Verification items for the finished model (mm, model axes). A direction names the side the tool comes from. Give positions to 0.01 mm unless a question says otherwise; leave off trailing zeros. Loops run counter-clockwise (first coordinate to the right, second up) from the corner with the lowest first, then second, coordinate; pieces in that order, holes last. Notation, with made-up numbers: (34.25, -9) - (87.25, -9) arc R21 cw to (87.25, 7) - close; hole circle Ø4 at (7, 86). An arc over 180 degrees is marked (long way). Use one line per item in the form item = value.
```python
from build123d import *

# Parameters (mm, degrees)
SKETCH068_R  = 1.7
PAD050_DEPTH = 100
SKETCH067_R  = 1.5
PAD049_DEPTH = 3
PAD048_DEPTH = 3


with BuildPart() as mountscrewcutouts:
    # Sketch068 → Pad050 (new body)
    with BuildSketch(Plane.XY):
        with Locations((28.75, 0)):
            Circle(SKETCH068_R)
        with Locations((18.75, 0)):
            Circle(SKETCH068_R)
    extrude(amount=-PAD050_DEPTH)


with BuildPart() as baseplate:
    # Sketch067 → Pad049 (new body)
    with BuildSketch(Plane(origin=(0, 0, -23), x_dir=(-1, 0, 0), z_dir=(0, 0, 1))):
        Polygon((-31.5, -4), (-31.5, 4), (-16.5, 7.5), (0, 7.5), (0, -7.5), (-16.5, -7.5), align=None)
        with Locations((-5, 3)):
            Circle(SKETCH067_R, mode=Mode.SUBTRACT)
        with Locations((-5, -3)):
            Circle(SKETCH067_R, mode=Mode.SUBTRACT)
    extrude(amount=-PAD049_DEPTH)


with BuildPart() as supportplate:
    # Sketch066 → Pad048 (new body)
    with BuildSketch(Plane(origin=(0, 0, -20), x_dir=(-1, 0, 0), z_dir=(0, 0, 1))):
        Polygon((-31.5, -4), (-31.5, 4), (-16.5, 7.5), (-16.5, -7.5), align=None)
    extrude(amount=-PAD048_DEPTH)

    # Fusion004017: union BasePlate
    add(baseplate.part)

    # Cut007017: cut MountScrewCutouts
    add(mountscrewcutouts.part, mode=Mode.SUBTRACT)


with BuildPart() as fusion004018:
    # Part__Mirroring001: instance of SupportPlate
    add(supportplate.part.mirror(Plane(origin=(0, 0, 0), x_dir=(0, -1, 0), z_dir=(1, 0, 0))))

    # Fusion004018: union SupportPlate
    add(supportplate.part)


solid = fusion004018.part
```
1. Tool access check on faces 5 (the flat face through (0, 0, -23)), 6 (the flat face through (-24, 0, -20)). Record the directions out of +Z, -Z, +X, -X, +Y, -Y that give a thin tool (end or side, any length) a straight path to the whole face; none if there is none.
Result set:
face_5 = +Z, +Y, -Y
face_6 = +Z, +X, -X, +Y, -Y
2. Section check B-B, the plane y = 3. Record the cut outline in (x, z).
Result set:
outline = (-31.5, -26) - (-6.5, -26) - (-6.5, -23) - (-16.5, -23) - (-16.5, -20) - (-31.5, -20) - close; (-3.5, -26) - (3.5, -26) - (3.5, -23) - (-3.5, -23) - close; (6.5, -26) - (31.5, -26) - (31.5, -20) - (16.5, -20) - (16.5, -23) - (6.5, -23) - close
3. Scan lines: probe 1 along X at (y, z) = (3, -24.15); probe 2 along X at (y, z) = (3, -20.7); probe 3 along Y at (x, z) = (4, -23.55). Record each from-to range of solid material in increasing order.
Result set:
probe_1 = -31.5 to -6.5, -3.5 to 3.5, 6.5 to 31.5
probe_2 = -31.5 to -16.5, 16.5 to 31.5
probe_3 = -7.5 to -4.12, -1.88 to 1.88, 4.12 to 7.5
4. Draft check along Y on faces 1 (the cylindrical face through (-20.3, -0.7, -23)), 2 (the flat face through (-16.5, 0, -21)), 3 (the flat face through (23.895, 5.774, -22.958)), 4 (the cylindrical face through (30.3, -0.7, -23)). Enter one of: released by +Y, released by -Y, zero draft, split by the parting line, or undercut.
Result set:
face_1 = undercut
face_2 = zero draft
face_3 = released by +Y
face_4 = undercut
5. Depth check by flat-ended pin: pin 1 Ø7.5 at (x, y) = (1.5, 1.5) entering from +Z. Enter the tip coordinate at first touch or a pass-through.
Result set:
pin_1 = -23
6. Section check C-C, the plane x = 5. Record the cut outline in (y, z), then the cut area to 3 significant figures.
Result set:
outline = (-7.5, -26) - (-4.5, -26) - (-4.5, -23) - (-7.5, -23) - close; (-1.5, -26) - (1.5, -26) - (1.5, -23) - (-1.5, -23) - close; (4.5, -26) - (7.5, -26) - (7.5, -23) - (4.5, -23) - close
area = 27.0 mm²
7. Section check D-D, the plane y = 0. Record the cut outline in (x, z), then the cut area to 3 significant figures.
Result set:
outline = (-31.5, -26) - (-30.45, -26) - (-30.45, -20) - (-31.5, -20) - close; (-27.05, -26) - (-20.45, -26) - (-20.45, -20) - (-27.05, -20) - close; (-17.05, -26) - (17.05, -26) - (17.05, -20) - (16.5, -20) - (16.5, -23) - (-16.5, -23) - (-16.5, -20) - (-17.05, -20) - close; (20.45, -26) - (27.05, -26) - (27.05, -20) - (20.45, -20) - close; (30.45, -26) - (31.5, -26) - (31.5, -20) - (30.45, -20) - close
area = 197 mm²
8. Section check A-A, the plane z = -20.85. Record the cut outline in (x, y), then the cut area to 3 significant figures.
Result set:
outline = (-31.5, -4) - (-16.5, -7.5) - (-16.5, 7.5) - (-31.5, 4) - close; (16.5, -7.5) - (31.5, -4) - (31.5, 4) - (16.5, 7.5) - close; hole circle Ø3.4 at (-28.75, 0); hole circle Ø3.4 at (-18.75, 0); hole circle Ø3.4 at (18.75, 0); hole circle Ø3.4 at (28.75, 0)
area = 309 mm²
